Could you check a few things on this model? Use its own coordinates, in mm. Face numbers are marked on the shaded views. A direction names the side the tool comes from. Round coordinates to 2 decimals unless told otherwise and drop trailing zeros. Loops run counter-clockwise (first coordinate to the right, second up) from the corner with the lowest first, then second, coordinate; pieces in that order, holes last. Notation, with made-up numbers: M -19.75,55.5 L 37.25,55.5 A17 ccw 37.25,66.5 Z; hole C 43,67.25 d10. An arc over 180 degrees is marked long. Return JSON: item names as keys, results as strings. Group by question number.
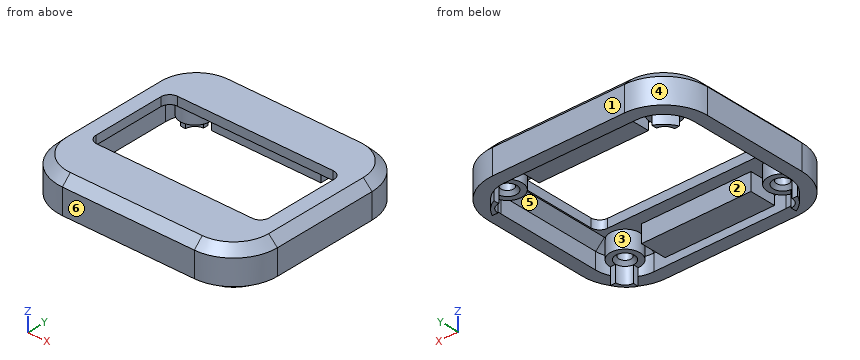
```python
from build123d import *

# Parameters (mm, degrees)
SKETCH1_W                = 39.55
SKETCH1_H                = 20.5
BOSS_EXTRUDE1_DEPTH      = 2
BOSS_EXTRUDE2_DEPTH      = 5.75
SKETCH3_W                = 25
SKETCH3_H                = 6
BOSS_EXTRUDE3_DEPTH      = 4
FILLET1_R                = 2
CHAMFER1_SIZE            = 2
CHAMFER2_SIZE            = 2
SKETCH4_R                = 3.4
SKETCH4_R_2              = 1.4
BOSS_EXTRUDE4_DEPTH      = 4
CHAMFER3_SIZE            = 0.75
CHAMFER3_OF_MIRROR1_SIZE = 0.75
BOSS_EXTRUDE6_DEPTH      = 3.75
MIRROR4_COPY_1_DEPTH     = 3.75


# Read off the part's stored shape, not the designer's step: Mirror2
with BuildPart() as part:
    # Sketch1 → Boss-Extrude1 (new body)
    with BuildSketch(Plane.XY.offset(57.451538964)):
        with BuildLine():
            Line((-141.643342382, 29.433342856), (-141.643342382, 5.333342856))
            ThreePointArc((-141.643342382, 5.333342856), (-138.714410194, -1.737724956), (-131.643342382, -4.666657144))
            Line((-131.643342382, -4.666657144), (-101.493342382, -4.666657144))
            ThreePointArc((-101.493342382, -4.666657144), (-94.42227457, -1.737724956), (-91.493342382, 5.333342856))
            Line((-91.493342382, 5.333342856), (-91.493342382, 29.433342856))
            ThreePointArc((-91.493342382, 29.433342856), (-94.42227457, 36.504410668), (-101.493342382, 39.433342856))
            Line((-101.493342382, 39.433342856), (-131.643342382, 39.433342856))
            ThreePointArc((-131.643342382, 39.433342856), (-138.714410194, 36.504410668), (-141.643342382, 29.433342856))
        make_face()
        with Locations((-116.568342382, 17.383342856)):
            Rectangle(SKETCH1_W, SKETCH1_H, mode=Mode.SUBTRACT)
    extrude(amount=-BOSS_EXTRUDE1_DEPTH)

    # Sketch2 → Boss-Extrude2 (add)
    with BuildSketch(Plane(origin=(0, 0, 55.451538964), x_dir=(-1, 0, 0), z_dir=(0, 0, -1))):
        with BuildLine():
            Line((141.643342382, 5.333342856), (141.643342382, 29.433342856))
            ThreePointArc((141.643342382, 29.433342856), (138.714410194, 36.504410668), (131.643342382, 39.433342856))
            Line((131.643342382, 39.433342856), (101.493342382, 39.433342856))
            ThreePointArc((101.493342382, 39.433342856), (94.42227457, 36.504410668), (91.493342382, 29.433342856))
            Line((91.493342382, 29.433342856), (91.493342382, 5.333342856))
            ThreePointArc((91.493342382, 5.333342856), (94.42227457, -1.737724956), (101.493342382, -4.666657144))
            Line((101.493342382, -4.666657144), (131.643342382, -4.666657144))
            ThreePointArc((131.643342382, -4.666657144), (138.714410194, -1.737724956), (141.643342382, 5.333342856))
        make_face()
        with BuildLine():
            Line((138.643342382, 5.333342856), (138.643342382, 29.433342856))
            ThreePointArc((138.643342382, 29.433342856), (136.59308985, 34.383090325), (131.643342382, 36.433342856))
            Line((131.643342382, 36.433342856), (101.493342382, 36.433342856))
            ThreePointArc((101.493342382, 36.433342856), (96.543594913, 34.383090325), (94.493342382, 29.433342856))
            Line((94.493342382, 29.433342856), (94.493342382, 5.333342856))
            ThreePointArc((94.493342382, 5.333342856), (96.543594913, 0.383595388), (101.493342382, -1.666657144))
            Line((101.493342382, -1.666657144), (131.643342382, -1.666657144))
            ThreePointArc((131.643342382, -1.666657144), (136.59308985, 0.383595388), (138.643342382, 5.333342856))
        make_face(mode=Mode.SUBTRACT)
    extrude(amount=BOSS_EXTRUDE2_DEPTH)

    # Sketch3 → Boss-Extrude3 (add)
    with BuildSketch(Plane(origin=(0, 0, 55.451538964), x_dir=(-1, 0, 0), z_dir=(0, 0, -1))):
        with Locations((116.568342382, 33.433342856)):
            Rectangle(SKETCH3_W, SKETCH3_H)
        with Locations((116.568342382, 1.333342856)):
            Rectangle(SKETCH3_W, SKETCH3_H)
    extrude(amount=BOSS_EXTRUDE3_DEPTH)

    # Fillet1
    fillet1_edges = [part.edges().sort_by_distance(p)[0] for p in [
        (-136.343342382, 27.633342856, 56.451538964),
        (-136.343342382, 7.133342856, 56.451538964),
        (-96.793342382, 7.133342856, 56.451538964),
        (-96.793342382, 27.633342856, 56.451538964),
    ]]
    fillet(fillet1_edges, radius=FILLET1_R)

    # Chamfer1
    chamfer1_edges = [part.edges().sort_by_distance(p)[0] for p in [
        (-138.714410194, 36.504410668, 57.451538964),
        (-116.568342382, 39.433342856, 57.451538964),
        (-94.42227457, 36.504410668, 57.451538964),
        (-91.493342382, 17.383342856, 57.451538964),
        (-94.42227457, -1.737724956, 57.451538964),
        (-116.568342382, -4.666657144, 57.451538964),
        (-138.714410194, -1.737724956, 57.451538964),
        (-141.643342382, 17.383342856, 57.451538964),
    ]]
    chamfer(chamfer1_edges, length=CHAMFER1_SIZE)

    # Chamfer2
    chamfer2_edges = [part.edges().sort_by_distance(p)[0] for p in [
        (-136.59308985, 0.383595388, 55.451538964),
        (-138.643342382, 17.383342856, 55.451538964),
        (-136.59308985, 34.383090325, 55.451538964),
        (-130.355842382, 36.433342856, 55.451538964),
        (-96.543594913, 34.383090325, 55.451538964),
        (-94.493342382, 17.383342856, 55.451538964),
        (-96.543594913, 0.383595388, 55.451538964),
        (-102.780842382, -1.666657144, 55.451538964),
        (-102.780842382, 36.433342856, 55.451538964),
        (-130.355842382, -1.666657144, 55.451538964),
    ]]
    chamfer(chamfer2_edges, length=CHAMFER2_SIZE)

    # Sketch4 → Boss-Extrude4 (add)
    with BuildSketch(Plane(origin=(0, 0, 55.451538964), x_dir=(-1, 0, 0), z_dir=(0, 0, -1))):
        with Locations((134.577835524, 32.367835998)):
            Circle(SKETCH4_R)
        with Locations(Location((134.577835524, 32.367835998, 0), (0, 0, 104.95728905))):
            Circle(SKETCH4_R_2, mode=Mode.SUBTRACT)
    boss_extrude4 = extrude(amount=BOSS_EXTRUDE4_DEPTH)

    # Chamfer3
    chamfer3_edges = [part.edges().sort_by_distance(p)[0] for p in [
        (-134.939174021, 31.015270107, 51.451538964),
    ]]
    chamfer(chamfer3_edges, length=CHAMFER3_SIZE)

    # Mirror1: Boss-Extrude4 across plane
    add(boss_extrude4.mirror(Plane(origin=(-116.568342382, 0, 0), x_dir=(0, 0, 1), z_dir=(1, 0, 0))))

    # Chamfer3 of Mirror1
    chamfer3_of_mirror1_edges = [part.edges().sort_by_distance(p)[0] for p in [
        (-98.197510742, 31.015270107, 51.451538964),
    ]]
    chamfer(chamfer3_of_mirror1_edges, length=CHAMFER3_OF_MIRROR1_SIZE)

    # Mirror2 outline → Mirror2 (revolve)
    with BuildSketch(Plane(origin=(-98.55884924, 2.398849714, 0), x_dir=(1, 0, 0), z_dir=(0, -1, 0))):
        Polygon((1.4, 52.201538964), (2.15, 51.451538964), (3.4, 51.451538964), (3.4, 55.451538967), (1.4, 55.451538967), align=None)
    revolve(axis=Axis((-98.55884924, 2.398849714, 0), (0, 0, 1)))

    # Mirror2 2 outline → Mirror2 2 (revolve)
    with BuildSketch(Plane(origin=(-134.577835524, 2.398849714, 0), x_dir=(1, 0, 0), z_dir=(0, -1, 0))):
        Polygon((1.4, 52.201538964), (2.15, 51.451538964), (3.4, 51.451538964), (3.4, 55.451538967), (1.4, 55.451538967), align=None)
    revolve(axis=Axis((-134.577835524, 2.398849714, 0), (0, 0, 1)))

    # Sketch5 → Boss-Extrude6 (add)
    with BuildSketch(Plane(origin=(0, 0, 51.451538964), x_dir=(-1, 0, 0), z_dir=(0, 0, -1))):
        with BuildLine():
            Line((98.55884924, 34.517835998), (98.513747348, 35.767536841))
            ThreePointArc((98.513747348, 35.767536841), (96.543594913, 34.383090325), (95.159148397, 32.41293789))
            Line((95.159148397, 32.41293789), (96.40884924, 32.367835998))
            ThreePointArc((96.40884924, 32.367835998), (97.03856966, 33.888115578), (98.55884924, 34.517835998))
        make_face()
    boss_extrude6 = extrude(amount=BOSS_EXTRUDE6_DEPTH)

    # Mirror3: Boss-Extrude6 across plane
    add(boss_extrude6.mirror(Plane(origin=(-116.568342382, 0, 0), x_dir=(0, 0, 1), z_dir=(1, 0, 0))))

    # Mirror4: Boss-Extrude6 across plane
    add(boss_extrude6.mirror(Plane.ZX.offset(17.383342856)))

    # Mirror4 copy 1 sketch → Mirror4 copy 1 (add)
    with BuildSketch(Plane(origin=(-233.136684763, 34.766685713, 51.451538964), x_dir=(1, 0, 0), z_dir=(0, 0, -1))):
        with BuildLine():
            Line((98.55884924, 34.517835998), (98.513747348, 35.767536841))
            ThreePointArc((98.513747348, 35.767536841), (96.543594913, 34.383090325), (95.159148397, 32.41293789))
            Line((95.159148397, 32.41293789), (96.40884924, 32.367835998))
            ThreePointArc((96.40884924, 32.367835998), (97.03856966, 33.888115578), (98.55884924, 34.517835998))
        make_face()
    extrude(amount=MIRROR4_COPY_1_DEPTH)


solid = part.part
```
1. If we section it at D-D, the plane z = 56.25: Please give me the cut outline in (x, y), then the cut area to 3 significant figures.
2. I need wall thicknesses on probe 1 along X at (y, z) = (18, 51); probe 2 along Y at (x, z) = (-134.5, 54); probe 3 along Y at (x, z) = (-126, 50.25). Which ranges of each line are inside material? Lowest first, please.
3. We'd pull the mould along X, two halves only. Please class the marked faces 1, 2, 3 and 4: +X half, -X half, draft (parallel to the pull), parting line (faces both ways), or undercut.
4. On a 3-axis mill with a long thin cutter (end or side, diameter ignored), from which of +Z, -Z, +X, -X, +Y, -Y can I reach the whole of each face in a straight line? I mean the marked faces 5 and 6. Say none if no direction works.
5. If we section it at A-A, the plane z = 48.75: Please give me the cut outline in (x, y).
6. I'm going to push flat-ended pins straight in: pin 1 Ø2 at (x, y) = (-98, 31) entering from -Z; pin 2 Ø3 at (x, y) = (-98.56, 2.4) entering from -Z; pin 3 Ø0.8 at (x, y) = (-134.5, 3) entering from -Z; pin 4 Ø2 at (x, y) = (-103, 9) entering from -Z. Where does each tip first touch, or does it pass through?
7. If we section it at B-B, the plane x = -119.5: Please give me the cut outline in (y, z), then the cut area to 3 significant figures.
8. If we section it at C-C, the plane y = 21: Please give me the cut outline in (x, z).
Geometry results:
{
 "1": {"outline": "M -140.84,5.33 A9.2 ccw -131.64,-3.87 L -101.49,-3.87 A9.2 ccw -92.29,5.33 L -92.29,29.43 A9.2 ccw -101.49,38.63 L -131.64,38.63 A9.2 ccw -140.84,29.43 Z; hole M -136.34,9.13 A2 ccw -134.34,7.13 L -98.79,7.13 A2 ccw -96.79,9.13 L -96.79,25.63 A2 ccw -98.79,27.63 L -134.34,27.63 A2 ccw -136.34,25.63 Z", "area": "1,180 mm^2"},
 "2": {"probe 1": "-141.64 to -138.64, -94.49 to -91.49", "probe 2": "-4.25 to 1, 3.8 to 5.8, 28.97 to 30.97, 33.77 to 39.02", "probe 3": "-4.67 to -1.67, 36.43 to 39.43"},
 "3": {"face 1": "draft", "face 2": "undercut", "face 3": "undercut", "face 4": "-X half"},
 "4": {"face 5": "-Z", "face 6": "+Z, -Z, +X, -X, -Y"},
 "5": {"outline": "M -137.98,2.35 A7 ccw -134.62,-1 L -134.58,0.25 A2.15 cw -136.73,2.4 Z; M -137.98,32.41 L -136.73,32.37 A2.15 cw -134.58,34.52 L -134.62,35.77 A7 ccw Z; M -98.56,0.25 L -98.51,-1 A7 ccw -95.16,2.35 L -96.41,2.4 A2.15 cw Z; M -98.56,34.52 A2.15 cw -96.41,32.37 L -95.16,32.41 A7 ccw -98.51,35.77 Z"},
 "6": {"pin 1": "z = 51.45", "pin 2": "z = 52.1", "pin 3": "z = 55.45", "pin 4": "through"},
 "7": {"outline": "M -4.67,49.7 L -1.67,49.7 L -1.67,51.45 L 4.33,51.45 L 4.33,55.45 L 7.13,55.45 L 7.13,57.45 L -2.67,57.45 L -4.67,55.45 Z; M 27.63,55.45 L 30.43,55.45 L 30.43,51.45 L 36.43,51.45 L 36.43,49.7 L 39.43,49.7 L 39.43,55.45 L 37.43,57.45 L 27.63,57.45 Z", "area": "126 mm^2"},
 "8": {"outline": "M -141.64,49.7 L -138.64,49.7 L -138.64,53.45 L -136.64,55.45 L -136.34,55.45 L -136.34,57.45 L -139.64,57.45 L -141.64,55.45 Z; M -96.79,55.45 L -96.49,55.45 L -94.49,53.45 L -94.49,49.7 L -91.49,49.7 L -91.49,55.45 L -93.49,57.45 L -96.79,57.45 Z"}
}
